```python
from build123d import *

# Parameters (mm, degrees)
SKETCH1_R           = 9
BOSS_EXTRUDE1_DEPTH = 34
SKETCH2_R           = 4
BOSS_EXTRUDE2_DEPTH = 1
FILLET1_R           = 1
CHAMFER1_SIZE       = 1


with BuildPart() as part:
    # Sketch1 → Boss-Extrude1 (new body)
    with BuildSketch(Plane(origin=(0, 0, 0), x_dir=(1, 0, 0), z_dir=(0, 1, 0))):
        with Locations(Location((0, 0, 0), (0, 0, 270))):
            Circle(SKETCH1_R)
    extrude(amount=BOSS_EXTRUDE1_DEPTH)

    # Sketch2 → Boss-Extrude2 (add)
    with BuildSketch(Plane(origin=(0, 34, 0), x_dir=(1, 0, 0), z_dir=(0, 1, 0))):
        with Locations(Location((0, 0, 0), (0, 0, 270))):
            Circle(SKETCH2_R)
    extrude(amount=BOSS_EXTRUDE2_DEPTH)

    # Fillet1
    fillet1_edges = [part.edges().sort_by_distance(p)[0] for p in [
        (0, 0, -9),
        (0, 34, -9),
    ]]
    fillet(fillet1_edges, radius=FILLET1_R)

    # Chamfer1
    chamfer1_edges = [part.edges().sort_by_distance(p)[0] for p in [
        (0, 34, -4),
    ]]
    chamfer(chamfer1_edges, length=CHAMFER1_SIZE - 0.0001)  # a hair under: the kernel refuses the full size


solid = part.part
```
CAD build for the part. Positions are in the model's coordinates, mm. A direction names the side the tool comes from. Coordinates: 2 decimals unless noted, no trailing zeros. Order: outer loops, then holes, each group sorted by start corner. A loop starts at its lowest first (then second) coordinate and runs counter-clockwise, first axis right, second up.
(1) Pin check, flat tips, straight feed: pin 1 Ø2 at (y, z) = (23.5, -7) entering from +X; pin 2 Ø6 at (x, y) = (-6.5, 23.5) entering from -Z; pin 3 Ø10 at (y, z) = (31, 6) entering from -X. Stop position of each tip, or through.
Solution:
pin 1: stops at x = 6.71
pin 2: stops at z = -8.29
pin 3: stops at x = -8.94
(2) Drill centre lines: L1, parallel to X at y = 10, z = 0.25; L2, parallel to Y at x = -5, z = -4.5; L3, parallel to X at y = 9, z = 6.5. Where is each one in solid material? Low to high.
Solution:
L1: x = -9 to 9
L2: y = 0 to 34
L3: x = -6.22 to 6.22
(3) Which spindle directions (+Z, -Z, +X, -X, +Y, -Y) get a long thin tool onto all of the face, cutting with end or side? Do faces 1 (the face through (2.703, 16.776, 8.584)), 2 (the face through (-5.2, 34, -0.1)). Say none if no direction does.
Solution:
face 1: +Y, -Y
face 2: +Y
(4) Saw through at C-C, the plane y = 7.5. Write the cut outline in (x, z).
Solution:
outline: circle Ø18 at (0, 0)
